Autodesk Inventor part; units mm, degrees
ref_plane "YZ Plane" through (0, 0, 0) normal (1, 0, 0) x (0, 1, 0)
ref_plane "XZ Plane" through (0, 0, 0) normal (0, 1, 0) x (-1, 0, 0)
ref_plane "XY Plane" through (0, 0, 0) normal (0, 0, 1) x (1, 0, 0)
sketch "Sketch1" plane through (0, 0, 0) normal (0, 1, 0) x (-1, 0, 0)
  circle A0 centre (0, 0) radius 73.025
  dimension "d0" = 146.05
extrude "Extrusion1" add sketch "Sketch1" along normal blind 254
sketch "Sketch2" plane through (0, 254, 0) normal (0, 1, 0) x (1, 0, 0)
  circle A0 centre (0, 0) radius 73.025
  circle A1 centre (0, 0) radius 71.4375
  dimension "d3" = 1.5875
extrude "Extrusion2" cut sketch "Sketch2" against normal blind 252.4125 contours A1
sketch "Sketch3" plane through (0, 0, 0) normal (0, -1, 0) x (1, 0, 0)
  circle A0 centre (0, 0) radius 73.025
  point P0 (0, 73.025)
ref_plane "Work Plane1" through (0, 0, 73.025) normal (0, 0, 1) x (1, 0, 0)
sketch "Sketch4" plane through (0, 0, 73.025) normal (0, 0, 1) x (1, 0, 0)
  circle A0 centre (0, 25.4) radius 3.175
  point P0 (0, 0)
  dimension "d6" = 6.35
  dimension "d7" = 25.4
extrude "Extrusion3" cut sketch "Sketch4" against normal blind 25.4
sketch "Sketch5" plane through (0, 1.5875, 0) normal (0, 1, 0) x (1, 0, 0)
  circle A0 centre (0, 0) radius 71.4375
  point P0 (0, -71.4375)
ref_plane "Work Plane2" through (0, 1.5875, 71.4375) normal (0, 0, 1) x (1, 0, 0)
sketch "Sketch6" plane through (0, 1.5875, 71.4375) normal (0, 0, 1) x (1, 0, 0)
  line L0 (-71.4375, 0) -> (71.4375, 0)
  line L1 (-71.4375, 252.4125) -> (71.4375, 252.4125)
  point P0 (0, -1.5875)
  point P1 (3.175, 23.8125)
  point P2 (0, 23.8125)
properties part number "Water Jug" material "PC/ABS Plastic"
Work out the finished part from the listing and answer in its coordinate system (mm). A direction names the side the tool comes from. Coordinates: 2 decimals unless noted, no trailing zeros. Order: outer loops, then holes, each group sorted by start corner. A loop starts at its lowest first (then second) coordinate and runs counter-clockwise, first axis right, second up. Notation, with made-up numbers: (71.25, 53) - (127.25, 53) arc R27 ccw to (127.25, 85) - close; hole circle Ø11 at (53, 59). An arc over 180 degrees is marked (long way). Put each result on its own line as item: value. Start each with the question number.
1) Find the intervals of material crossed by line 1 (Y direction, x = 0, z = 72.7) (3 decimals); line 2 (Z direction, x = 0, y = 90) (1 decimal); line 3 (Y direction, x = -36, z = -7), in increasing order. Write a range as from..to.
2) Find section A-A (x = 0). Give the vertices of the cut face in (y, z) (1 decimal), plus the area to 3 significant figures.
3) For a pull along X with two mould halves and no side action, classify faces 3 (the cylindrical face through (-0.41, 28.55, 72.21)), 4 (the flat face through (1, 0, 1)), 5 (the cylindrical face through (-69.653, 125.222, -21.935)) as released by +X, released by -X, zero draft, split by the parting line, or undercut.
4) Find section B-B (z = 60.5). Give the vertices of the cut face in (x, y) (1 decimal), plus the area to 3 significant figures.
5) For faces 1 (the flat face through (-54, 254, -48)), 2 (the cylindrical face through (-71.37, 129.56, -3.14)), determine the directions among +Z, -Z, +X, -X, +Y, -Y from which every point of the face is accessible in a straight line to the end or side of a thin tool.
6) Flat-ended cylindrical pins translate along their axes: pin 1 (2 mm diameter, centred on y = 44.5, z = 4.5, fed in from -X); pin 2 (3 mm diameter, centred on x = 33, y = 78, fed in from +Z); pin 3 (1.5 mm diameter, centred on x = 25, z = 42, fed in from +Y). Find the tip coordinate at first contact, or state that the pin passes through.
7) Find section D-D (x = -26.5). Give the vertices of the cut face in (y, z), plus the area to 3 significant figures.
Results list:
1. line 1: y = 0..22.225, 28.575..254
1. line 2: z = -73..-71.4, 71.4..73
1. line 3: y = 0..1.59
2. outline: (0, -73) - (254, -73) - (254, -71.4) - (1.6, -71.4) - (1.6, 71.4) - (22.2, 71.4) - (22.2, 73) - (0, 73) - close; (28.6, 71.4) - (254, 71.4) - (254, 73) - (28.6, 73) - close
2. area: 1,020 mm^2
3. face 3: undercut
3. face 4: zero draft
3. face 5: split by the parting line
4. outline: (-40.9, 0) - (40.9, 0) - (40.9, 254) - (38, 254) - (38, 1.6) - (-38, 1.6) - (-38, 254) - (-40.9, 254) - close
4. area: 1,600 mm^2
5. face 1: +Z, -Z, +X, -X, +Y
5. face 2: +Y
6. pin 1: stops at x = -72.94
6. pin 2: stops at z = 65.88
6. pin 3: stops at y = 1.59
7. outline: (0, -68.05) - (254, -68.05) - (254, -66.34) - (1.59, -66.34) - (1.59, 66.34) - (254, 66.34) - (254, 68.05) - (0, 68.05) - close
7. area: 1,080 mm^2
